from build123d import *

# Parameters (mm, degrees)
F0_R     = 2.15
F1_DEPTH = 5
F2_W     = 60
F2_H     = 3
F3_DEPTH = 20
F5_DEPTH = 4
F6_DEPTH = 60
F8_DEPTH = 3


# Not quite as in the source:
# - a feature names something its author has since deleted; it is built from what else it names


with BuildPart() as f1:
    # F0 (on Top) → F1 (new body)
    with BuildSketch(Plane.XY):
        with BuildLine():
            ThreePointArc((-10, 4.6267989092), (-9.5606601718, 5.6874590809), (-8.5, 6.1267989092))
            Line((-8.5, 6.1267989092), (-30, 6.1267989092))
            Line((-30, 6.1267989092), (-30, -16.8732010908))
            Line((-30, -16.8732010908), (30, -16.8732010908))
            Line((30, -16.8732010908), (30, 6.1267989092))
            Line((30, 6.1267989092), (8.4999999793, 6.1267989092))
            ThreePointArc((8.4999999793, 6.1267989092), (9.5606601645, 5.6874590882), (10, 4.6267989092))
            ThreePointArc((10, 4.6267989092), (0, -5.3732010908), (-10, 4.6267989092))
        make_face()
        with Locations((-21.3480107486, -5.3732010908)):
            Circle(F0_R, mode=Mode.SUBTRACT)
        with Locations((21.3480107486, -5.3732010908)):
            Circle(F0_R, mode=Mode.SUBTRACT)
        with BuildLine():
            ThreePointArc((-7, 4.6267989092), (-7.4393398282, 5.6874590809), (-8.5, 6.1267989092))
            ThreePointArc((-8.5, 6.1267989092), (-9.5606601718, 5.6874590809), (-10, 4.6267989092))
            ThreePointArc((-10, 4.6267989092), (0, -5.3732010908), (10, 4.6267989092))
            ThreePointArc((10, 4.6267989092), (9.5606601645, 5.6874590882), (8.4999999793, 6.1267989092))
            ThreePointArc((8.4999999793, 6.1267989092), (7.4393398209, 5.6874590736), (7, 4.6267989092))
            ThreePointArc((7, 4.6267989092), (0, -2.3732010908), (-7, 4.6267989092))
        make_face()
        with BuildLine():
            Line((8, 6.1267989092), (-8, 6.1267989092))
            Line((-8, 6.1267989092), (-8.5, 6.1267989092))
            ThreePointArc((-8.5, 6.1267989092), (-7.4393398282, 5.6874590809), (-7, 4.6267989092))
            ThreePointArc((-7, 4.6267989092), (0, -2.3732010908), (7, 4.6267989092))
            ThreePointArc((7, 4.6267989092), (7.4393398209, 5.6874590736), (8.4999999793, 6.1267989092))
            Line((8.4999999793, 6.1267989092), (8, 6.1267989092))
        make_face()
    extrude(amount=F1_DEPTH)

    # F2 (on face) → F3 (join)
    with BuildSketch(Plane.XY.offset(5)):
        with Locations((0, 4.6267989092)):
            Rectangle(F2_W, F2_H)
    extrude(amount=F3_DEPTH)

    # F4 (on face) → F5 (cut)
    with BuildSketch(Plane.XZ.offset(-3.1267989092)):
        with BuildLine():
            Line((-30, 25), (-30, 13))
            ThreePointArc((-30, 13), (-21.5147186258, 16.5147186258), (-18, 25))
            Line((-18, 25), (-30, 25))
        make_face()
        with BuildLine():
            Line((30, 25), (18, 25))
            ThreePointArc((18, 25), (21.5147186258, 16.5147186258), (30, 13))
            Line((30, 13), (30, 25))
        make_face()
    extrude(amount=-F5_DEPTH, mode=Mode.SUBTRACT)

    # F0 (on Top) → F6 (join)
    with BuildSketch(Plane.XY):
        with BuildLine():
            ThreePointArc((-7, 4.6267989092), (-7.4393398282, 5.6874590809), (-8.5, 6.1267989092))
            ThreePointArc((-8.5, 6.1267989092), (-9.5606601718, 5.6874590809), (-10, 4.6267989092))
            ThreePointArc((-10, 4.6267989092), (0, -5.3732010908), (10, 4.6267989092))
            ThreePointArc((10, 4.6267989092), (9.5606601645, 5.6874590882), (8.4999999793, 6.1267989092))
            ThreePointArc((8.4999999793, 6.1267989092), (7.4393398209, 5.6874590736), (7, 4.6267989092))
            ThreePointArc((7, 4.6267989092), (0, -2.3732010908), (-7, 4.6267989092))
        make_face()
    extrude(amount=-F6_DEPTH)

    # F7 (on face) → F8 (join)
    with BuildSketch(Plane(origin=(0, 0, -60), x_dir=(1, 0, 0), z_dir=(0, 0, -1))):
        with BuildLine():
            ThreePointArc((20, -4.6267989092), (0, 15.3732010908), (-20, -4.6267989092))
            Line((-20, -4.6267989092), (-10, -4.6267989092))
            ThreePointArc((-10, -4.6267989092), (0, 5.3732010908), (10, -4.6267989092))
            Line((10, -4.6267989092), (20, -4.6267989092))
        make_face()
        with BuildLine():
            ThreePointArc((10, -4.6267989092), (0, 5.3732010908), (-10, -4.6267989092))
            Line((-10, -4.6267989092), (-7, -4.6267989092))
            ThreePointArc((-7, -4.6267989092), (0, 2.3732010908), (7, -4.6267989092))
            Line((7, -4.6267989092), (10, -4.6267989092))
        make_face()
    extrude(amount=-F8_DEPTH)


solid = f1.part
Here's how the part is built. I have some questions about the finished solid (model axes, mm). A direction names the side the tool comes from. Round coordinates to 2 decimals unless told otherwise and drop trailing zeros. Loops run counter-clockwise (first coordinate to the right, second up) from the corner with the lowest first, then second, coordinate; pieces in that order, holes last.
1. We'd pull the mould along Y, two halves only. Please class faces 1 (the face through (0, -5, -60)), 2 (the face through (23.4, -4.73, 2.46)), 3 (the face through (0.15, -2.37, -29.58)), 4 (the face through (0, 3.127, 13)): +Y half, -Y half, draft (parallel to the pull), parting line (faces both ways), or undercut.
Answer list:
face 1: draft
face 2: undercut
face 3: +Y half
face 4: -Y half
2. If I drill on line 1 along X through (y, z) = (4.75, -42.5); line 2 along Z through (x, y) = (-15.5, 2); line 3 along Y through (x, z) = (-19, 6), over which ranges is the centre line in solid material (lowest first)?
Answer list:
line 1: x = -9.99 to -7.01, 7.01 to 9.99
line 2: z = -60 to -57, 0 to 5
line 3: y = 3.13 to 6.13
3. If we section it at A-A on x = -15: Write out the boundary of the cut face in (y, z).
Answer list:
outline: (-16.87, 0) - (6.13, 0) - (6.13, 25) - (3.13, 25) - (3.13, 5) - (-16.87, 5) - close; (-8.6, -60) - (4.63, -60) - (4.63, -57) - (-8.6, -57) - close
4. If we section it at C-C on z = -22: Write out the boundary of the cut face in (x, y), plus the area to 3 significant figures.
Answer list:
outline: (-10, 4.63) arc R10 ccw to (10, 4.63) arc R1.5 ccw to (7, 4.63) arc R7 cw to (-7, 4.63) arc R1.5 ccw to start
area: 87.2 mm2
5. Which directions (+Z, -Z, +X, -X, +Y, -Y) give clear straight access to the entire face, cutting with the end or side of a thin tool? Please do faces 5 (the face through (0, -7, 5)), 6 (the face through (15, 4.627, -59)), 7 (the face through (0.44, -15.37, -58.52)).
Answer list:
face 5: +Z, +X, -X, -Y
face 6: -Z, +X, +Y
face 7: -Z, -Y
6. For P1, Ø6, axis at y = -2, z = -21, coming from the -X side; P2, Ø2.5, axis at x = 15, z = -58, coming from the +Y side; P3, Ø7, axis at x = 21.35, y = -5.37, coming from the +Z side, each with a flat end and sliding along its axis, tell me the tip position at first contact or that it passes through.
Answer list:
P1: stops at x = -9.32
P2: stops at y = 4.63
P3: stops at z = 5
7. If we section it at D-D on x = 0: Write out the boundary of the cut face in (y, z), plus the area to 3 significant figures.
Answer list:
outline: (-16.87, 0) - (-5.37, 0) - (-5.37, -57) - (-15.37, -57) - (-15.37, -60) - (-2.37, -60) - (-2.37, 0) - (6.13, 0) - (6.13, 25) - (3.13, 25) - (3.13, 5) - (-16.87, 5) - close
area: 385 mm2
8. If we section it at B-B on y = -9.25: Write out the boundary of the cut face in (x, z).
Answer list:
outline: (-30, 0) - (30, 0) - (30, 5) - (-30, 5) - close; (-14.4, -60) - (14.4, -60) - (14.4, -57) - (-14.4, -57) - close
